from build123d import *

# Parameters (mm, degrees)
SKETCH_1_W      = 25
SKETCH_1_H      = 30
SKETCH_1_R      = 1.3
SKETCH_1_R_2    = 3.05
EXTRUDE_1_DEPTH = 1.6


with BuildPart() as part:
    # 草图1 → 凸台-拉伸1 (new body)
    with BuildSketch(Plane.XY):
        with Locations((12.5, 15)):
            Rectangle(SKETCH_1_W, SKETCH_1_H)
        with Locations((4.368272016, 20.631727984)):
            Circle(SKETCH_1_R, mode=Mode.SUBTRACT)
        with Locations(Location((20.631727984, 20.631727984, 0), (0, 0, 180))):
            Circle(SKETCH_1_R, mode=Mode.SUBTRACT)
        with Locations((20.631727984, 4.368272016)):
            Circle(SKETCH_1_R, mode=Mode.SUBTRACT)
        with Locations(Location((4.368272016, 4.368272016, 0), (0, 0, 180))):
            Circle(SKETCH_1_R, mode=Mode.SUBTRACT)
        with Locations((12.5, 12.5)):
            Circle(SKETCH_1_R_2, mode=Mode.SUBTRACT)
    extrude(amount=EXTRUDE_1_DEPTH)


solid = part.part
Can you work these out from the model? Positions are in its coordinate system, mm. Give positions to 0.01 mm unless a question says otherwise; leave off trailing zeros. Loops run counter-clockwise (first coordinate to the right, second up) from the corner with the lowest first, then second, coordinate; pieces in that order, holes last. Notation, with made-up numbers: M 81,43.5 L 134,43.5 A34 cw 134,79.5 Z; hole C 6.5,57 d9. An arc over 180 degrees is marked long. One line per item, written item: value. Start each with the question number.
1) If we section it at A-A, the plane x = 12.5: Write out the boundary of the cut face in (y, z), and give its area (3 significant figures).
2) Thinking about a two-plate mould opening in Y: for faces 1 (the face through (12, 0, 1)), 2 (the face through (4.65, 5.637, 0.789)), 3 (the face through (10, 15, 0)), which applies, +Y half, -Y half, draft (parallel to the pull), parting line (faces both ways), or undercut?
3) If we section it at C-C, the plane y = 5.25: Write out the boundary of the cut face in (x, z), and give its area (3 significant figures).
4) If we section it at B-B, the plane y = 12.5: Write out the boundary of the cut face in (x, z), and give its area (3 significant figures).
5) If I drill on line 1 (Y direction, x = 4.5, z = 1.45); line 2 (Y direction, x = 12.5, z = 1.25); line 3 (Y direction, x = 10.75, z = 1.3), over which ranges is the centre line in solid material (lowest first)? Write a range as [from, to].
6) If we section it at D-D, the plane x = 5: Write out the boundary of the cut face in (y, z).
Completed:
1. outline: M 0,0 L 9.45,0 L 9.45,1.6 L 0,1.6 Z; M 15.55,0 L 30,0 L 30,1.6 L 15.55,1.6 Z
1. area: 38.2 mm^2
2. face 1: -Y half
2. face 2: undercut
2. face 3: draft
3. outline: M 0,0 L 3.41,0 L 3.41,1.6 L 0,1.6 Z; M 5.32,0 L 19.68,0 L 19.68,1.6 L 5.32,1.6 Z; M 21.59,0 L 25,0 L 25,1.6 L 21.59,1.6 Z
3. area: 33.9 mm^2
4. outline: M 0,0 L 9.45,0 L 9.45,1.6 L 0,1.6 Z; M 15.55,0 L 25,0 L 25,1.6 L 15.55,1.6 Z
4. area: 30.2 mm^2
5. line 1: y = [0, 3.07], [5.66, 19.34], [21.93, 30]
5. line 2: y = [0, 9.45], [15.55, 30]
5. line 3: y = [0, 10], [15, 30]
6. outline: M 0,0 L 3.23,0 L 3.23,1.6 L 0,1.6 Z; M 5.5,0 L 19.5,0 L 19.5,1.6 L 5.5,1.6 Z; M 21.77,0 L 30,0 L 30,1.6 L 21.77,1.6 Z
